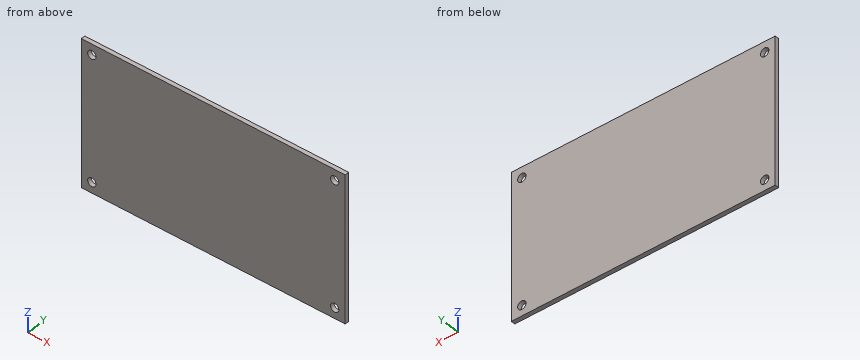
from build123d import *

# Parameters (mm, degrees)
SKETCH1_W           = 200
SKETCH1_H           = 110
BOSS_EXTRUDE1_DEPTH = 3.175
CUT_EXTRUDE1_REACH  = 5.175
SKETCH2_R           = 3.175


with BuildPart() as part:
    # Sketch1 → Boss-Extrude1 (new body)
    with BuildSketch(Plane(origin=(0, 0, 0), x_dir=(1, 0, 0), z_dir=(0, 1, 0))):
        with Locations((100, 55)):
            Rectangle(SKETCH1_W, SKETCH1_H)
    extrude(amount=BOSS_EXTRUDE1_DEPTH)

    # Sketch2 → Cut-Extrude1 (cut, up to next)
    with BuildSketch(Plane(origin=(0, 3.175, 0), x_dir=(1, 0, 0), z_dir=(0, 1, 0)), mode=Mode.PRIVATE) as cut_extrude1_sk1:
        with Locations((8, 102)):
            Circle(SKETCH2_R)
    cut_extrude1_tool1 = extrude(cut_extrude1_sk1.sketch, amount=-CUT_EXTRUDE1_REACH, mode=Mode.PRIVATE) & part.part
    add(cut_extrude1_tool1.solids().sort_by_distance((8, 3.175, -102))[0], mode=Mode.SUBTRACT)
    # Sketch2 → Cut-Extrude1 (cut, up to next)
    with BuildSketch(Plane(origin=(0, 3.175, 0), x_dir=(1, 0, 0), z_dir=(0, 1, 0)), mode=Mode.PRIVATE) as cut_extrude1_sk2:
        with Locations((192, 102)):
            Circle(SKETCH2_R)
    cut_extrude1_tool2 = extrude(cut_extrude1_sk2.sketch, amount=-CUT_EXTRUDE1_REACH, mode=Mode.PRIVATE) & part.part
    add(cut_extrude1_tool2.solids().sort_by_distance((192, 3.175, -102))[0], mode=Mode.SUBTRACT)
    # Sketch2 → Cut-Extrude1 (cut, up to next)
    with BuildSketch(Plane(origin=(0, 3.175, 0), x_dir=(1, 0, 0), z_dir=(0, 1, 0)), mode=Mode.PRIVATE) as cut_extrude1_sk3:
        with Locations((192, 8)):
            Circle(SKETCH2_R)
    cut_extrude1_tool3 = extrude(cut_extrude1_sk3.sketch, amount=-CUT_EXTRUDE1_REACH, mode=Mode.PRIVATE) & part.part
    add(cut_extrude1_tool3.solids().sort_by_distance((192, 3.175, -8))[0], mode=Mode.SUBTRACT)
    # Sketch2 → Cut-Extrude1 (cut, up to next)
    with BuildSketch(Plane(origin=(0, 3.175, 0), x_dir=(1, 0, 0), z_dir=(0, 1, 0)), mode=Mode.PRIVATE) as cut_extrude1_sk4:
        with Locations((8, 8)):
            Circle(SKETCH2_R)
    cut_extrude1_tool4 = extrude(cut_extrude1_sk4.sketch, amount=-CUT_EXTRUDE1_REACH, mode=Mode.PRIVATE) & part.part
    add(cut_extrude1_tool4.solids().sort_by_distance((8, 3.175, -8))[0], mode=Mode.SUBTRACT)


solid = part.part
Model file for the job. Use its own axes, mm. Give positions to 0.01 mm unless a question says otherwise; leave off trailing zeros. Loops run counter-clockwise (first coordinate to the right, second up) from the corner with the lowest first, then second, coordinate; pieces in that order, holes last. Notation, with made-up numbers: (-18.5, 40.25) - (39.5, 40.25) arc R17 cw to (39.5, 44.25) - close; hole circle Ø9 at (32.5, -15). An arc over 180 degrees is marked (long way). Use one line per item in the form item = value.
(1) Cut at A-A (x = 192). Give the cut face in (y, z) (3 decimals), then the cut area to 3 significant figures.
Determined:
outline = (0, -110) - (3.175, -110) - (3.175, -105.175) - (0, -105.175) - close; (0, -98.825) - (3.175, -98.825) - (3.175, -11.175) - (0, -11.175) - close; (0, -4.825) - (3.175, -4.825) - (3.175, 0) - (0, 0) - close
area = 309 mm^2
(2) Drill centre lines: L1, parallel to Z at x = 8, y = 1.5 (3 decimals); L2, parallel to X at y = 2.3, z = -8 (3 decimals); L3, parallel to Z at x = 191.5, y = 0.4. Where is each one in solid material? Low to high.
Determined:
L1 = -110 to -105.175, -98.825 to -11.175, -4.825 to 0
L2 = 0 to 4.825, 11.175 to 188.825, 195.175 to 200
L3 = -110 to -105.14, -98.86 to -11.14, -4.86 to 0
(3) Drop a flat-ended pin along its axis: P1, Ø5.5, axis at x = 192, z = -8, coming from the -Y side. Give the stop position or say it passes through.
Determined:
P1 = through
(4) Cut at B-B (z = -102). Give the cut face in (x, y) (3 decimals).
Determined:
outline = (0, 0) - (4.825, 0) - (4.825, 3.175) - (0, 3.175) - close; (11.175, 0) - (188.825, 0) - (188.825, 3.175) - (11.175, 3.175) - close; (195.175, 0) - (200, 0) - (200, 3.175) - (195.175, 3.175) - close
